Could you check a few things on this model? Use its own coordinates, in mm. A direction names the side the tool comes from. Coordinates: 2 decimals unless noted, no trailing zeros. Loops run counter-clockwise (first coordinate to the right, second up) from the corner with the lowest first, then second, coordinate; pieces in that order, holes last. Notation, with made-up numbers: M -9.5,12.5 L 13.5,12.5 A10 ccw 13.5,19.5 Z; hole C 63.25,39 d10. An arc over 180 degrees is marked long. Use one line per item in the form item = value. Start each with the question number.
```python
from build123d import *

# Parameters (mm, degrees)
F1_DEPTH = 23


with BuildPart() as f1:
    # F0 (on Top) → F1 (new body)
    with BuildSketch(Plane.XY):
        Polygon((-27, 2.207249), (-27, -2.792751), (27, -2.792751), (27, 2.207249), (17.565055, 2.207249), (12.565055, 2.207249), (6.050185, 2.207249), (3.317844, 0), (-6.682156, 0), (-7.026023, 0), (-7.026023, 5), (-12.444239, 0), (-22.444239, 0), (-22.444239, 10), align=None)
        Polygon((12.565055, 2.207249), (17.565055, 2.207249), (26.487442, 30.849717), (21.487442, 30.849717), align=None)
    extrude(amount=F1_DEPTH)


solid = f1.part
```
Item 1: I'm going to push flat-ended pins straight in: P1, Ø4, axis at x = -20, y = 13, coming from the -Z side; P2, Ø2, axis at x = -21, z = 19.5, coming from the +Y side; P3, Ø8, axis at y = 11.5, z = 18.5, coming from the -X side; P4, Ø2, axis at y = 27, z = 17.5, coming from the -X side. Where does each tip first touch, or does it pass through?
Item 2: For faces 4 (the flat face through (-17, 0, 11)), 5 (the flat face through (22, 2.207, 11)), 6 (the flat face through (-27, 0, 11)), which set-ups out of +Z, -Z, +X, -X, +Y, -Y let a thin tool reach every point of the face, with its end or its side?
Item 3: Thinking about a two-plate mould opening in Y: for faces 1 (the flat face through (8, 2, 23)), 2 (the flat face through (-2, 0, 11)), 3 (the flat face through (21.964, 16.328, 11.339)), which applies, pulls with the +Y half, pulls with the -Y half, needs draft (parallel to the pull), parting line crosses it, or undercut?
Item 4: I want a section at A-A (z = 20.25). Write out the boundary of the cut face in (x, y), plus the area to 3 significant figures.
Item 5: I want a section at B-B (x = 18.5). Write out the boundary of the cut face in (y, z), plus the area to 3 significant figures.
Item 6: I want a section at D-D (y = 13.5). Write out the boundary of the cut face in (x, z), plus the area to 3 significant figures.
Item 7: Please list where these lines run through material, in increasing order: line 1 along X through (y, z) = (1.5, 14); line 2 along Y through (x, z) = (-3.5, 19); line 3 along Y through (x, z) = (8, 8.75).
Item 8: I want a section at C-C (x = -16). Write out the boundary of the cut face in (y, z), plus the area to 3 significant figures.
Worked answers:
q1.P1 = through
q1.P2 = 0
q1.P3 = -23.91
q1.P4 = 19.98
q2.face_4 = +Z, -Z, +Y
q2.face_5 = +Z, -Z, +X
q2.face_6 = +Z, -Z, -X, +Y, -Y
q3.face_1 = needs draft
q3.face_2 = pulls with the +Y half
q3.face_3 = undercut
q4.outline = M -27,-2.79 L 27,-2.79 L 27,2.21 L 17.57,2.21 L 26.49,30.85 L 21.49,30.85 L 12.57,2.21 L 6.05,2.21 L 3.32,0 L -7.03,0 L -7.03,5 L -12.44,0 L -22.44,0 L -22.44,10 L -27,2.21 Z
q4.area = 385 mm²
q5.outline = M -2.79,0 L 2.21,0 L 2.21,23 L -2.79,23 Z; M 5.21,0 L 21.26,0 L 21.26,23 L 5.21,23 Z
q5.area = 484 mm²
q6.outline = M 16.08,0 L 21.08,0 L 21.08,23 L 16.08,23 Z
q6.area = 115 mm²
q7.line_1 = -27 to -22.44, -10.82 to -7.03, 5.17 to 27
q7.line_2 = -2.79 to 0
q7.line_3 = -2.79 to 2.21
q8.outline = M -2.79,0 L 0,0 L 0,23 L -2.79,23 Z
q8.area = 64.2 mm²
